For this review, take the finished solid that the model builds, in its own axes (mm). A direction names the side the tool comes from. Coordinates: 2 decimals unless noted, no trailing zeros. Loops run counter-clockwise (first coordinate to the right, second up) from the corner with the lowest first, then second, coordinate; pieces in that order, holes last. Notation, with made-up numbers: M 1.5,35.5 L 26.5,35.5 A34 cw 26.5,67.5 Z; hole C 32,73 d6. An arc over 180 degrees is marked long. Use one line per item in the form item = value.
```python
from build123d import *

# Parameters (mm, degrees)
SKETCH1_W               = 56.35
SKETCH1_H               = 16.8
BOSS_EXTRUDE1_DEPTH     = 1.5
SKETCH2_R               = 1
CUT_EXTRUDE1_DEPTH      = 30.438760589
MIRROR2_COPY_1_SKETCH_R = 1
MIRROR2_COPY_1_DEPTH    = 30.438760589
FILLET1_R               = 1
BOSS_EXTRUDE2_DEPTH     = 7.5
SKETCH4_W               = 18.8
SKETCH4_H               = 15.8
BOSS_EXTRUDE3_DEPTH     = 7.5


with BuildPart() as part:
    # Sketch1 → Boss-Extrude1 (new body)
    with BuildSketch(Plane(origin=(0, 0, 0), x_dir=(1, 0, 0), z_dir=(0, 1, 0))):
        Rectangle(SKETCH1_W, SKETCH1_H)
    extrude(amount=BOSS_EXTRUDE1_DEPTH)

    # Sketch2 → Cut-Extrude1 (cut, through all)
    with BuildSketch(Plane(origin=(0, 1.5, 0), x_dir=(1, 0, 0), z_dir=(0, 1, 0))):
        with Locations(Location((-26.675, 6.9, 0), (0, 0, 270))):
            Circle(SKETCH2_R)
    cut_extrude1 = extrude(amount=-CUT_EXTRUDE1_DEPTH, mode=Mode.SUBTRACT)

    # Mirror1: Cut-Extrude1 across plane
    add(cut_extrude1.mirror(Plane.XY), mode=Mode.SUBTRACT)

    # Mirror2: Cut-Extrude1 across plane
    add(cut_extrude1.mirror(Plane(origin=(0, 0, 0), x_dir=(0, 0, 1), z_dir=(1, 0, 0))), mode=Mode.SUBTRACT)

    # Mirror2 copy 1 sketch → Mirror2 copy 1 (cut, through all)
    with BuildSketch(Plane(origin=(0, 1.5, 0), x_dir=(-1, 0, 0), z_dir=(0, 1, 0))):
        with Locations(Location((-26.675, 6.9, 0), (0, 0, 270))):
            Circle(MIRROR2_COPY_1_SKETCH_R)
    extrude(amount=-MIRROR2_COPY_1_DEPTH, mode=Mode.SUBTRACT)

    # Fillet1
    fillet1_edges = [part.edges().sort_by_distance(p)[0] for p in [
        (28.175, 0.75, 8.4),
        (-28.175, 0.75, 8.4),
        (-28.175, 0.75, -8.4),
        (28.175, 0.75, -8.4),
    ]]
    fillet(fillet1_edges, radius=FILLET1_R)

    # Sketch3 → Boss-Extrude2 (add, symmetric)
    with BuildSketch(Plane.XY):
        Polygon((18.775, 11.5), (17.375, 7.5), (17.375, 1.5), (25.175, 1.5), (25.175, 7.5), (23.775, 11.5), align=None)
    boss_extrude2 = extrude(amount=BOSS_EXTRUDE2_DEPTH, both=True)

    # Mirror3: Boss-Extrude2 across plane
    add(boss_extrude2.mirror(Plane(origin=(0, 0, 0), x_dir=(0, 0, 1), z_dir=(1, 0, 0))))

    # Sketch4 → Boss-Extrude3 (add, symmetric)
    with BuildSketch(Plane.XY):
        with Locations((-7.875, 9.4)):
            Rectangle(SKETCH4_W, SKETCH4_H)
    extrude(amount=BOSS_EXTRUDE3_DEPTH, both=True)


solid = part.part
```
1. Consider section C-C on x = -23. Write out the cut boundary in (y, z).
Computed values:
outline = M 0,-8.4 L 1.5,-8.4 L 1.5,-7.5 L 11.5,-7.5 L 11.5,7.5 L 1.5,7.5 L 1.5,8.4 L 0,8.4 Z
2. Consider section B-B on z = -6.9. Write out the cut boundary in (x, y) (3 decimals).
Computed values:
outline = M -28.175,0 L -27.675,0 L -27.675,1.5 L -28.175,1.5 Z; M -25.675,0 L 25.675,0 L 25.675,1.5 L 25.175,1.5 L 25.175,7.5 L 23.775,11.5 L 18.775,11.5 L 17.375,7.5 L 17.375,1.5 L 1.525,1.5 L 1.525,17.3 L -17.275,17.3 L -17.275,1.5 L -17.375,1.5 L -17.375,7.5 L -18.775,11.5 L -23.775,11.5 L -25.175,7.5 L -25.175,1.5 L -25.675,1.5 Z; M 27.675,0 L 28.175,0 L 28.175,1.5 L 27.675,1.5 Z
3. Consider section A-A on y = 2.25. Write out the cut boundary in (x, z) (3 decimals).
Computed values:
outline = M -25.175,-7.5 L -17.375,-7.5 L -17.375,7.5 L -25.175,7.5 Z; M -17.275,-7.5 L 1.525,-7.5 L 1.525,7.5 L -17.275,7.5 Z; M 17.375,-7.5 L 25.175,-7.5 L 25.175,7.5 L 17.375,7.5 Z
4. Consider section D-D on z = -4.75. Write out the cut boundary in (x, y) (3 decimals).
Computed values:
outline = M -28.175,0 L 28.175,0 L 28.175,1.5 L 25.175,1.5 L 25.175,7.5 L 23.775,11.5 L 18.775,11.5 L 17.375,7.5 L 17.375,1.5 L 1.525,1.5 L 1.525,17.3 L -17.275,17.3 L -17.275,1.5 L -17.375,1.5 L -17.375,7.5 L -18.775,11.5 L -23.775,11.5 L -25.175,7.5 L -25.175,1.5 L -28.175,1.5 Z
5. Draft analysis for pull direction X (two halves, no side actions). For faces 4 (the face through (1.525, 9, 0)), 5 (the face through (-24.485, 9.472, 0.105)), 6 (the face through (-21, 7, 7.5)), state which applies: +X half, -X half, draft (parallel to the pull), parting line (faces both ways), or undercut.
Computed values:
face_4 = undercut
face_5 = -X half
face_6 = draft
6. Tool access review of faces 1 (the face through (21, 7, 7.5)), 2 (the face through (21, 11.5, 0)), 3 (the face through (-21, 11.5, 0)): name each direction out of +Z, -Z, +X, -X, +Y, -Y from which nothing blocks a thin tool from reaching the whole face with its end or side.
Computed values:
face_1 = +Z, +X, -X, +Y
face_2 = +Z, -Z, +X, +Y
face_3 = +Z, -Z, -X, +Y
7. For pin 1 Ø1.6 at (x, z) = (26.675, 6.9) entering from +Y; pin 2 Ø4.5 at (x, y) = (-5, 10.5) entering from -Z; pin 3 Ø5 at (y, z) = (6, 0.5) entering from +X (3 decimals); pin 4 Ø4.5 at (y, z) = (10, -3) entering from -X, all flat-tipped, find the tip position at first contact; note any pin that passes through.
Computed values:
pin_1 = through
pin_2 = -7.5
pin_3 = 25.175
pin_4 = -25.09
8. Wall thickness on line 1 along X through (y, z) = (0.6, 6.9) (3 decimals); line 2 along X through (y, z) = (9, -5.25) (3 decimals); line 3 along Y through (x, z) = (11, 6.25): over which ranges is each line inside the solid? List them lowest first. Write a range as from..to.
Computed values:
line_1 = -28.175..-27.675, -25.675..25.675, 27.675..28.175
line_2 = -24.65..-17.9, -17.275..1.525, 17.9..24.65
line_3 = 0..1.5
